Part model, mm, in its own coordinate system. A direction names the side the tool comes from. Give positions to 0.01 mm unless a question says otherwise; leave off trailing zeros. Write each loop counter-clockwise with the first axis right and the second up, starting at its lowest first coordinate (ties: lowest second). Pieces come first, ordered by that corner, then holes. Notation, with made-up numbers: (-25.75, 37) - (-15.75, 37) arc R30 ccw to (-15.75, 59) - close; hole circle Ø5 at (-26.75, 67.25). An arc over 180 degrees is marked (long way). Answer as a JSON object with one key per item and string values. Group by question number.
```python
from build123d import *

# Parameters (mm, degrees)
F0_R     = 2.3919393617
F1_DEPTH = 7.9375
F2_R     = 3.0192979406
F2_R_2   = 2.3919393617
F2_R_3   = 3.0900236713
F2_R_4   = 3.0639016039
F2_R_5   = 3.0180013539
F2_R_6   = 3.0358198122
F3_DEPTH = 0.79375
F4_R     = 3.0946781872
F4_R_2   = 2.3919393617
F4_R_3   = 3.0440395285
F4_R_4   = 3.0438317033
F4_R_5   = 3.080942185
F4_R_6   = 2.996685824
F5_DEPTH = 0.79375


with BuildPart() as f1:
    # F0 (on Top) → F1 (new body)
    with BuildSketch(Plane.XY):
        with BuildLine():
            ThreePointArc((-3.1748391564, 6.3618900805), (-0.0650994939, 3.8236435926), (-1.9082323266, 0.2576882701))
            ThreePointArc((-1.9082323266, 0.2576882701), (-0.4943758214, 1.4282223533), (0.0359294434, 3.1854692293))
            ThreePointArc((0.0359294434, 3.1854692293), (-0.9065879549, 5.443714368), (-3.1748391564, 6.3618900805))
        make_face()
        with BuildLine():
            ThreePointArc((-36.5301852994, 5.9214270067), (-38.0657970886, 2.7730759979), (-35.7714141925, 0.1261863575))
            ThreePointArc((-35.7714141925, 0.1261863575), (-38.0245779178, 2.7784728257), (-36.5301852994, 5.9214270067))
        make_face()
        with BuildLine():
            ThreePointArc((-26.6891774485, 6.35), (-26.9658751282, 6.362073801), (-27.2425728079, 6.35))
            Line((-27.2425728079, 6.35), (-26.6891774485, 6.35))
        make_face()
        with BuildLine():
            Line((-19.2923728079, 6.35), (-18.7389774485, 6.35))
            ThreePointArc((-18.7389774485, 6.35), (-19.0156751282, 6.362073801), (-19.2923728079, 6.35))
        make_face()
        with BuildLine():
            Line((-11.3548728079, 6.35), (-10.8014774485, 6.35))
            ThreePointArc((-10.8014774485, 6.35), (-11.0781751282, 6.362073801), (-11.3548728079, 6.35))
        make_face()
        with BuildLine():
            Line((-34.594617784, 0), (-3.4232600592, 0))
            ThreePointArc((-3.4232600592, 0), (-2.6499734267, 0.0361112438), (-1.9082323266, 0.2576882701))
            ThreePointArc((-1.9082323266, 0.2576882701), (-6.2510268672, 2.54007891), (-3.1748391564, 6.3618900805))
            ThreePointArc((-3.1748391564, 6.3618900805), (-3.3171702803, 6.3591232625), (-3.4592356533, 6.35))
            Line((-3.4592356533, 6.35), (-10.8014774485, 6.35))
            ThreePointArc((-10.8014774485, 6.35), (-8.7361913838, 5.331611989), (-7.9015705566, 3.1854692293))
            ThreePointArc((-7.9015705566, 3.1854692293), (-13.224317888, 0.8434854848), (-11.3548728079, 6.35))
            Line((-11.3548728079, 6.35), (-18.7389774485, 6.35))
            ThreePointArc((-18.7389774485, 6.35), (-16.6736913838, 5.331611989), (-15.8390705566, 3.1854692293))
            ThreePointArc((-15.8390705566, 3.1854692293), (-21.161817888, 0.8434854848), (-19.2923728079, 6.35))
            Line((-19.2923728079, 6.35), (-26.6891774485, 6.35))
            ThreePointArc((-26.6891774485, 6.35), (-24.6238913838, 5.331611989), (-23.7892705566, 3.1854692293))
            ThreePointArc((-23.7892705566, 3.1854692293), (-29.112017888, 0.8434854848), (-27.2425728079, 6.35))
            Line((-27.2425728079, 6.35), (-34.2893563211, 6.35))
            ThreePointArc((-34.2893563211, 6.35), (-35.4492032163, 6.3418890662), (-36.5301852994, 5.9214270067))
            ThreePointArc((-36.5301852994, 5.9214270067), (-33.3407296335, 5.9439295203), (-31.7394705566, 3.1854692293))
            ThreePointArc((-31.7394705566, 3.1854692293), (-32.9959523948, 0.6548674643), (-35.7714141925, 0.1261863575))
            ThreePointArc((-35.7714141925, 0.1261863575), (-35.1888922767, 0.0082917303), (-34.594617784, 0))
        make_face()
        with BuildLine():
            ThreePointArc((-36.5301852994, 5.9214270067), (-38.0245779178, 2.7784728257), (-35.7714141925, 0.1261863575))
            ThreePointArc((-35.7714141925, 0.1261863575), (-32.9959523948, 0.6548674643), (-31.7394705566, 3.1854692293))
            ThreePointArc((-31.7394705566, 3.1854692293), (-33.3407296335, 5.9439295203), (-36.5301852994, 5.9214270067))
        make_face()
        with Locations((-34.9160751282, 3.1854692293)):
            Circle(F0_R, mode=Mode.SUBTRACT)
        with BuildLine():
            Line((-26.6891774485, 6.35), (-27.2425728079, 6.35))
            ThreePointArc((-27.2425728079, 6.35), (-29.112017888, 0.8434854848), (-23.7892705566, 3.1854692293))
            ThreePointArc((-23.7892705566, 3.1854692293), (-24.6238913838, 5.331611989), (-26.6891774485, 6.35))
        make_face()
        with Locations((-26.9658751282, 3.1854692293)):
            Circle(F0_R, mode=Mode.SUBTRACT)
        with BuildLine():
            ThreePointArc((-15.8390705566, 3.1854692293), (-16.6736913838, 5.331611989), (-18.7389774485, 6.35))
            Line((-18.7389774485, 6.35), (-19.2923728079, 6.35))
            ThreePointArc((-19.2923728079, 6.35), (-21.161817888, 0.8434854848), (-15.8390705566, 3.1854692293))
        make_face()
        with Locations((-19.0156751282, 3.1854692293)):
            Circle(F0_R, mode=Mode.SUBTRACT)
        with BuildLine():
            ThreePointArc((-7.9015705566, 3.1854692293), (-8.7361913838, 5.331611989), (-10.8014774485, 6.35))
            Line((-10.8014774485, 6.35), (-11.3548728079, 6.35))
            ThreePointArc((-11.3548728079, 6.35), (-13.224317888, 0.8434854848), (-7.9015705566, 3.1854692293))
        make_face()
        with Locations((-11.0781751282, 3.1854692293)):
            Circle(F0_R, mode=Mode.SUBTRACT)
        with BuildLine():
            ThreePointArc((-3.1748391564, 6.3618900805), (-6.2510268672, 2.54007891), (-1.9082323266, 0.2576882701))
            ThreePointArc((-1.9082323266, 0.2576882701), (-0.0650994939, 3.8236435926), (-3.1748391564, 6.3618900805))
        make_face()
        with Locations((-3.1406751282, 3.1854692293)):
            Circle(F0_R, mode=Mode.SUBTRACT)
    extrude(amount=F1_DEPTH)

    # F2 (on face) → F3 (cut)
    with BuildSketch(Plane.XY.offset(7.9375)):
        with Locations((-3.1406751282, 3.1854692293)):
            Circle(F2_R)
        with Locations((-3.1406751282, 3.1854692293)):
            Circle(F2_R_2, mode=Mode.SUBTRACT)
        with Locations((-11.0781751282, 3.1854692293)):
            Circle(F2_R_3)
        with Locations((-11.0781751282, 3.1854692293)):
            Circle(F2_R_2, mode=Mode.SUBTRACT)
        with Locations((-19.0156751282, 3.1854692293)):
            Circle(F2_R_4)
        with Locations((-19.0156751282, 3.1854692293)):
            Circle(F2_R_2, mode=Mode.SUBTRACT)
        with Locations((-26.9658751282, 3.1854692293)):
            Circle(F2_R_5)
        with Locations((-26.9658751282, 3.1854692293)):
            Circle(F2_R_2, mode=Mode.SUBTRACT)
        with Locations((-34.9160751282, 3.1854692293)):
            Circle(F2_R_6)
        with Locations((-34.9160751282, 3.1854692293)):
            Circle(F2_R_2, mode=Mode.SUBTRACT)
    extrude(amount=-F3_DEPTH, mode=Mode.SUBTRACT)

    # F4 (on face) → F5 (cut)
    with BuildSketch(Plane(origin=(0, 0, 0), x_dir=(1, 0, 0), z_dir=(0, 0, -1))):
        with Locations((-34.8472412506, -3.1944816519)):
            Circle(F4_R)
        with Locations((-34.9160751282, -3.1854692293)):
            Circle(F4_R_2, mode=Mode.SUBTRACT)
        with Locations((-26.9658751282, -3.1854692293)):
            Circle(F4_R_3)
        with Locations((-26.9658751282, -3.1854692293)):
            Circle(F4_R_2, mode=Mode.SUBTRACT)
        with Locations((-19.0156751282, -3.1854692293)):
            Circle(F4_R_4)
        with Locations((-19.0156751282, -3.1854692293)):
            Circle(F4_R_2, mode=Mode.SUBTRACT)
        with Locations((-11.0781751282, -3.1854692293)):
            Circle(F4_R_5)
        with Locations((-11.0781751282, -3.1854692293)):
            Circle(F4_R_2, mode=Mode.SUBTRACT)
        with Locations((-3.1406751282, -3.1854692293)):
            Circle(F4_R_6)
        with Locations((-3.1406751282, -3.1854692293)):
            Circle(F4_R_2, mode=Mode.SUBTRACT)
    extrude(amount=-F5_DEPTH, mode=Mode.SUBTRACT)


solid = f1.part
```
1) Which spindle directions (+Z, -Z, +X, -X, +Y, -Y) get a long thin tool onto all of the face, cutting with end or side? Do faces 1 (the flat face through (-5, 5, 7.144)), 2 (the flat face through (-15, 3, 7.938)), 3 (the flat face through (-9, 5, 0.794)), 4 (the cylindrical face through (-29.356, 3.291, 3.924)). Say none if no direction does.
2) Two-plate mould, pull along X, no slides. Class faces 5 (the flat face through (-29, 5, 7.144)), 6 (the cylindrical face through (-35.433, 6.345, 3.913)), 7 (the flat face through (-15, 3, 0)): +X half, -X half, draft (parallel to the pull), parting line (faces both ways), or undercut.
3) Drill centre lines: line 1 along X through (y, z) = (4.75, 7.75); line 2 along X through (y, z) = (1, 4.25); line 3 along Y through (x, z) = (-6, 3.75). Where is each one in solid material? Low to high. Write a range as from..to.
4) Saw through at B-B (z = 7.5). List the corners of the cut face in (x, y), and give its area (3 significant figures).
5) Saw through at A-A (x = -4). List the corners of the cut face in (y, z).
6) Drop flat-ended pins along their axis: P1, Ø3, axis at x = -10.5, z = 2.5, coming from the +Y side; P2, Ø3, axis at x = -35.5, y = 4, coming from the -Z side; P3, Ø2, axis at x = -16, z = 3.5, coming from the +Y side; P4, Ø1, axis at x = -20.5, y = 5.5, coming from the +Z side. Give the stop position or say it passes through.
7) Saw through at C-C (y = 1.25). State how many separate pieces and enclosed holes the cut face has, and give its area (3 significant figures).
Checks:
{
 "1": {"face 1": "+Z", "face 2": "+Z, +X, -X, +Y, -Y", "face 3": "-Z", "face 4": "+Z, -Z"},
 "2": {"face 5": "undercut", "face 6": "parting line", "face 7": "draft"},
 "3": {"line 1": "-37.68..-37.52, -32.31..-29.55, -24.39..-21.65, -16.38..-13.74, -8.41..-5.72, -0.56..-0.38", "line 2": "-37.22..-35.89, -33.94..-27.94, -25.99..-19.99, -18.04..-12.05, -10.11..-4.11, -2.17..-0.84", "line 3": "0..6.35"},
 "4": {"outline": "(-36.53, 5.92) arc R3.18 ccw to (-35.77, 0.13) arc R3.2 ccw to (-34.59, 0) - (-3.42, 0) arc R3.19 ccw to (-1.91, 0.26) arc R3.18 ccw to (-3.17, 6.36) arc R3.19 ccw to (-3.46, 6.35) - (-10.8, 6.35) arc R3.18 ccw to (-11.35, 6.35) - (-18.74, 6.35) arc R3.18 ccw to (-19.29, 6.35) - (-26.69, 6.35) arc R3.18 ccw to (-27.24, 6.35) - (-34.29, 6.35) arc R3.2 ccw to start; hole circle Ø6.07 at (-34.92, 3.19); hole circle Ø6.04 at (-26.97, 3.19); hole circle Ø6.13 at (-19.02, 3.19); hole circle Ø6.18 at (-11.08, 3.19); hole circle Ø6.04 at (-3.14, 3.19)", "area": "87.9 mm2"},
 "5": {"outline": "(0, 0) - (0.31, 0) - (0.31, 0.79) - (0.95, 0.79) - (0.95, 7.14) - (0.29, 7.14) - (0.29, 7.94) - (0, 7.94) - close; (5.42, 0.79) - (6.06, 0.79) - (6.06, 0) - (6.35, 0) - (6.35, 7.94) - (6.08, 7.94) - (6.08, 7.14) - (5.42, 7.14) - close"},
 "6": {"P1": "y = 6.36", "P2": "z = 0.79", "P3": "y = 6.35", "P4": "z = 7.94"},
 "7": {"separate pieces": "6", "enclosed holes": "0", "area": "166 mm2"}
}
